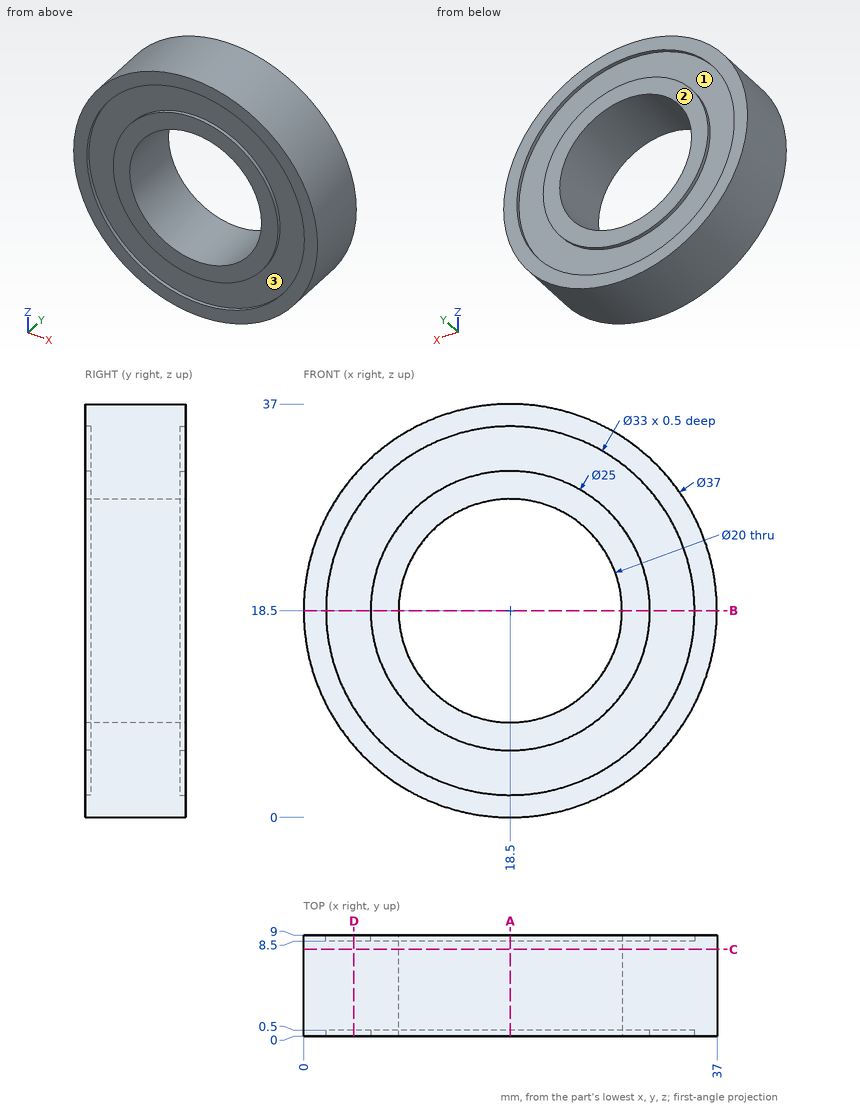
Part print with two shaded views. Sizes in mm from the minimum x, y, z corner. A direction names the side the tool comes from. Coordinates: 2 decimals unless noted, no trailing zeros. Loops run counter-clockwise (first coordinate to the right, second up) from the corner with the lowest first, then second, coordinate; pieces in that order, holes last. Notation, with made-up numbers: (10.25, -13) -> (27.25, -13) arc R26 ccw to (27.25, 19) -> close; hole circle Ø4 at (19, 18.25). An arc over 180 degrees is marked (long way). Answer as a JSON object with one key per item and string values.
Q1. Flat gauge pins, fed straight in: P1, Ø12, axis at x = 18.5, z = 18.5, coming from the +Y side; P2, Ø1.5, axis at y = 1.5, z = 30.5, coming from the -X side; P3, Ø4, axis at x = 21, y = 8, coming from the -Z side; P4, Ø4, axis at x = 22.5, y = 6, coming from the -Z side. Where does each tip first touch, or does it go through?
Report:
{"P1": "passes through", "P2": "stops at x = 3.81", "P3": "stops at z = 0.01", "P4": "stops at z = 0.11"}
Q2. Probe probe 1 along Z at (x, y) = (18.5, 8.85); probe 2 along Z at (x, y) = (18.5, 6.75); probe 3 along Y at (x, z) = (19.5, 34.5). List the from-to ranges inside material, lowest first.
Report:
{"probe 1": "z = 0 to 2, 6 to 8.5, 28.5 to 31, 35 to 37", "probe 2": "z = 0 to 8.5, 28.5 to 37", "probe 3": "y = 0.5 to 8.5"}
Q3. Cut at D-D (x = 4.5). List the corners of the cut face in (y, z).
Report:
{"outline": "(0, 6.41) -> (9, 6.41) -> (9, 9.77) -> (8.5, 9.77) -> (8.5, 27.23) -> (9, 27.23) -> (9, 30.59) -> (0, 30.59) -> (0, 27.23) -> (0.5, 27.23) -> (0.5, 9.77) -> (0, 9.77) -> close"}
Q4. Cut at A-A (x = 18.5). List the corners of the cut face in (y, z), and give its area (3 significant figures).
Report:
{"outline": "(0, 0) -> (9, 0) -> (9, 2) -> (8.5, 2) -> (8.5, 6) -> (9, 6) -> (9, 8.5) -> (0, 8.5) -> (0, 6) -> (0.5, 6) -> (0.5, 2) -> (0, 2) -> close; (0, 28.5) -> (9, 28.5) -> (9, 31) -> (8.5, 31) -> (8.5, 35) -> (9, 35) -> (9, 37) -> (0, 37) -> (0, 35) -> (0.5, 35) -> (0.5, 31) -> (0, 31) -> close", "area": "145 mm2"}
Q5. Cut at B-B (z = 18.5). List the corners of the cut face in (x, y).
Report:
{"outline": "(0, 0) -> (2, 0) -> (2, 0.5) -> (6, 0.5) -> (6, 0) -> (8.5, 0) -> (8.5, 9) -> (6, 9) -> (6, 8.5) -> (2, 8.5) -> (2, 9) -> (0, 9) -> close; (28.5, 0) -> (31, 0) -> (31, 0.5) -> (35, 0.5) -> (35, 0) -> (37, 0) -> (37, 9) -> (35, 9) -> (35, 8.5) -> (31, 8.5) -> (31, 9) -> (28.5, 9) -> close"}
Q6. Cut at C-C (y = 7.75). List the corners of the cut face in (x, z), and give its area (3 significant figures).
Report:
{"outline": "circle Ø37 at (18.5, 18.5); hole circle Ø20 at (18.5, 18.5)", "area": "761 mm2"}
Q7. 3-axis set-ups, long thin cutter, end or side, ignore diameter. For the marked faces 1, 2 and 3: which of +Z, -Z, +X, -X, +Y, -Y reach the whole face in a straight line?
Report:
{"face 1": "+Y", "face 2": "+Z, -Z, +X, -X, +Y", "face 3": "-Y"}
